The model under review builds one solid part; all positions refer to its coordinate system, in mm. Face numbers are marked on the shaded views. A direction names the side the tool comes from. Give positions to 0.01 mm unless a question says otherwise; leave off trailing zeros. Write each loop counter-clockwise with the first axis right and the second up, starting at its lowest first coordinate (ties: lowest second). Pieces come first, ordered by that corner, then holes. Notation, with made-up numbers: (77, 6.5) - (105, 6.5) arc R13 cw to (105, 12.5) - close; hole circle Ø10 at (39, 81.25). An arc over 180 degrees is marked (long way). One line per question, with ' | ' between items. Start each with the question number.
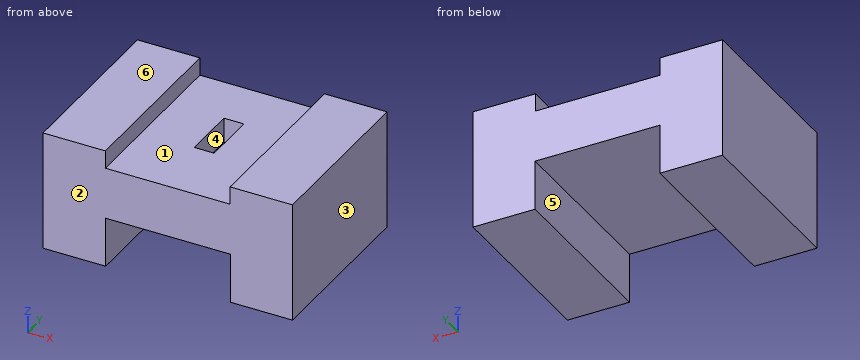
Autodesk Inventor part; units mm, degrees
ref_plane "YZ Plane" through (0, 0, 0) normal (1, 0, 0) x (0, 1, 0)
ref_plane "XZ Plane" through (0, 0, 0) normal (0, 1, 0) x (-1, 0, 0)
ref_plane "XY Plane" through (0, 0, 0) normal (0, 0, 1) x (1, 0, 0)
sketch "Sketch1" plane through (0, 0, 0) normal (0, 0, 1) x (1, 0, 0)
  line L0 (-117.1316, 93.6595) -> (132.8684, 93.6595)
  line L1 (132.8684, 93.6595) -> (132.8684, -81.3405)
  line L2 (132.8684, -81.3405) -> (-117.1316, -81.3405)
  line L3 (-117.1316, -81.3405) -> (-117.1316, 93.6595)
  line L4 (-54.6316, 93.6595) -> (-54.6316, -81.3405)
  line L5 (70.3684, 93.6595) -> (70.3684, -81.3405)
  line L6 (-27.1316, 41.1595) -> (42.8684, 41.1595)
  line L7 (42.8684, 41.1595) -> (42.8684, -28.8405)
  line L8 (42.8684, -28.8405) -> (-27.1316, -28.8405)
  line L9 (-27.1316, -28.8405) -> (-27.1316, 41.1595)
  circle A0 centre (7.8684, 18.6595) radius 10
  line L10 (-2.1316, 41.1595) -> (17.8684, 41.1595)
  line L11 (17.8684, 41.1595) -> (17.8684, -13.8405)
  line L12 (17.8684, -13.8405) -> (-2.1316, -13.8405)
  line L13 (-2.1316, -13.8405) -> (-2.1316, 41.1595)
  point P0 (17.8684, 41.1595)
  point P1 (17.8684, 18.6595)
  point P2 (-2.1316, 18.6595)
  dimension "d0" = 250
  dimension "d1" = 175
  dimension "d2" = 62.5
  dimension "d3" = 62.5
  dimension "d8" = 70
  dimension "d9" = 70
  dimension "d10" = 52.5
  dimension "d11" = 27.5
  dimension "d12" = 20
  dimension "d19" = 20
  dimension "d20" = 55
  dimension "d21" = 25
extrude "Extrusion1" add sketch "Sketch1" along normal blind 40 and the other way blind 80 contours L0 L4 L2 L3 | L0 L1 L2 L5
extrude "Extrusion2" add sketch "Sketch1" along normal blind 22 and the other way blind 80 contours L0 L5 L2 L4 | L6 L13 L12 L11 L7 L8 L9 | L6 L11 A0 L13 | A0 | A0 L11 L12 L13
extrude "Extrusion3" cut sketch "Sketch1" along normal blind 22 and the other way blind 3 contours L6 L11 A0 L13 | A0 | A0 L11 L12 L13
extrude "Extrusion4" cut sketch "Sketch1" against normal blind 25 contours A0
sketch "Sketch3" plane through (-117.1316, -81.3405, -80) normal (0, -1, 0) x (1, 0, 0)
  line L0 (0, 0) -> (250, 0)
  line L1 (62.8423, 0) -> (187.8423, 0)
  line L2 (187.8423, 0) -> (187.8423, 50)
  line L3 (187.8423, 50) -> (62.8423, 50)
  line L4 (62.8423, 50) -> (62.8423, 0)
  point P0 (117.1316, 80)
  dimension "d22" = 125
  dimension "d23" = 50
extrude "Extrusion5" cut sketch "Sketch3" against normal through all
equation "\"d0\" = 5 * Product_dia"
equation "\"d1\" = 3.5 * Product_dia"
equation "\"d2\" = 0.25 * d0"
equation "\"d3\" = d2"
equation "\"d10\" = -0.5 * d9 + 0.5 * d1"
equation "\"d11\" = -0.5 * d8 + 0.5 * d0 - d2"
equation "\"d21\" = -0.5 * d19 + 0.5 * d8"
equation "\"ProductBaseHeight\" = 35"
equation "\"GridClearance\" = 3"
equation "\"GridBorderThickness\" = 5"
equation "\"GridTotalSize\" = 63"
equation "\"GridBorderFillets\" = 7"
equation "\"BaseTotalWidth\" = 352"
equation "\"GridProcutClearance\" = 3"
Item 1: Take a section at B-B (y = -27). Give the boundary of the cut face in (x, z), plus the area to 3 significant figures.
Item 2: Take a section at A-A (z = -56.5). Give the boundary of the cut face in (x, y).
Item 3: Machinability: for the marked faces 4, 5 and 6, which of the approach directions +Z, -Z, +X, -X, +Y, -Y give a long, thin tool a straight path to every point of the face, cutting with its end or side? Answer none if there is none.
Item 4: The part is to be moulded in two halves that separate along X. For the marked faces 1, 2 and 3, say which applies: +X half, -X half, draft (parallel to the pull), parting line (faces both ways), or undercut.
Item 5: Take a section at C-C (x = 14). Give the boundary of the cut face in (y, z), plus the area to 3 significant figures.
Item 6: Clearance check with flat-ended pins moving along their axes: P1, Ø5, axis at x = 14, y = 25.5, coming from the -Z side; P2, Ø5, axis at x = -41.5, y = -31, coming from the +Z side. State where each tip first meets the part, or that it passes through.
Item 7: For probe 1 along X at (y, z) = (71, -62); probe 2 along X at (y, z) = (-11, 25.5); probe 3 along Z at (x, y) = (15.5, 76), list the stretches that pass through material, from the lowest coordinate up.
Item 8: Take a section at D-D (y = 35). Give the boundary of the cut face in (x, z).
Check sheet entries:
1) outline: (-117.13, -80) - (-54.29, -80) - (-54.29, -30) - (70.71, -30) - (70.71, -80) - (132.87, -80) - (132.87, 40) - (70.37, 40) - (70.37, 22) - (-54.63, 22) - (-54.63, 40) - (-117.13, 40) - close | area: 21,500 mm^2
2) outline: (-117.13, -81.34) - (-54.29, -81.34) - (-54.29, 93.66) - (-117.13, 93.66) - close; (70.71, -81.34) - (132.87, -81.34) - (132.87, 93.66) - (70.71, 93.66) - close
3) face 4: +Z | face 5: -Z, +Y, -Y | face 6: +Z, +X, -X, +Y, -Y
4) face 1: undercut | face 2: draft | face 3: +X half
5) outline: (-81.34, -30) - (93.66, -30) - (93.66, 22) - (41.16, 22) - (41.16, -3) - (26.56, -3) - (26.56, -25) - (10.76, -25) - (10.76, -3) - (-13.84, -3) - (-13.84, 22) - (-81.34, 22) - close | area: 7,380 mm^2
6) P1: stops at z = -30 | P2: stops at z = 22
7) probe 1: x = -117.13 to -54.29, 70.71 to 132.87 | probe 2: x = -117.13 to -54.63, 70.37 to 132.87 | probe 3: z = -30 to 22
8) outline: (-117.13, -80) - (-54.29, -80) - (-54.29, -30) - (70.71, -30) - (70.71, -80) - (132.87, -80) - (132.87, 40) - (70.37, 40) - (70.37, 22) - (17.87, 22) - (17.87, -3) - (-2.13, -3) - (-2.13, 22) - (-54.63, 22) - (-54.63, 40) - (-117.13, 40) - close
